```python
from build123d import *

# Parameters (mm, degrees)
SKETCH1_R           = 2.5
BOSS_EXTRUDE1_DEPTH = 3
SKETCH2_R           = 1.5
CUT_EXTRUDE1_DEPTH  = 77.127156728
FILLET1_R           = 10
SKETCH3_R           = 6
CUT_EXTRUDE2_DEPTH  = 77.127156728
BOSS_EXTRUDE3_DEPTH = 5
FILLET3_START       = -3.356502253
FILLET3_DEPTH       = 38.004734531
FILLET3_START_2     = -6
FILLET3_2_DEPTH     = 6


with BuildPart() as part:
    # Sketch1 → Boss-Extrude1 (new body)
    with BuildSketch(Plane.XY):
        with BuildLine():
            Line((0, -19), (30, -19))
            Line((30, -19), (64.201367261, 15.201367261))
            Line((64.201367261, 15.201367261), (58.615223689, 20.787510832))
            Line((58.615223689, 20.787510832), (44.190245353, 35.212489168))
            Line((44.190245353, 35.212489168), (38.604101782, 40.798632739))
            Line((38.604101782, 40.798632739), (16.805469042, 19))
            Line((16.805469042, 19), (0, 19))
            ThreePointArc((0, 19), (-19, 0), (0, -19))
        make_face()
        Circle(SKETCH1_R, mode=Mode.SUBTRACT)
    extrude(amount=BOSS_EXTRUDE1_DEPTH)

    # Sketch2 → Cut-Extrude1 (cut, through all)
    with BuildSketch(Plane.XY.offset(3)):
        with Locations((38.878105659, 35.574881393)):
            Circle(SKETCH2_R)
        with Locations((58.977615915, 15.475371138)):
            Circle(SKETCH2_R)
    extrude(amount=-CUT_EXTRUDE1_DEPTH, mode=Mode.SUBTRACT)

    # Fillet1
    fillet1_edges = [part.edges().sort_by_distance(p)[0] for p in [
        (16.805469042, 19, 1.5),
        (30, -19, 1.5),
    ]]
    fillet(fillet1_edges, radius=FILLET1_R)

    # Sketch3 → Cut-Extrude2 (cut, through all)
    with BuildSketch(Plane.XY.offset(3)):
        Circle(SKETCH3_R)
        Polygon((38.604101782, 40.798632739), (31.53303397, 33.727564928), (57.130299449, 8.130299449), (64.201367261, 15.201367261), align=None)
    extrude(amount=-CUT_EXTRUDE2_DEPTH, mode=Mode.SUBTRACT)

    # Sketch5 → Boss-Extrude3 (add)
    with BuildSketch(Plane(origin=(0, 0, 0), x_dir=(-1, 0, 0), z_dir=(0, 0, -1))):
        Polygon((-57.130299449, 8.130299449), (-31.53303397, 33.727564928), (-20.926432252, 23.12096321), (-46.523697731, -2.476302269), align=None)
    extrude(amount=BOSS_EXTRUDE3_DEPTH)

    # Fillet3: read off the stored shape, not the designer's step
    # Fillet3 outline → Fillet3 (add)
    with BuildSketch(Plane(origin=(0, 0, 0), x_dir=(0.707106781186548, 0.707106781186547, 0), z_dir=(0.707106781186547, -0.707106781186548, 0)).offset(FILLET3_START)):
        with BuildLine():
            ThreePointArc((23.730013537, 0), (28.202149492, -1.366750419), (31.146212025, -5))
            Line((31.146212025, -5), (31.146212025, 0))
            Line((31.146212025, 0), (23.730013537, 0))
        make_face()
    extrude(amount=FILLET3_DEPTH)

    # Fillet3 2 outline → Fillet3 2 (cut)
    with BuildSketch(Plane.XY.offset(FILLET3_START_2)):
        with BuildLine():
            Line((19.650292227, 24.397103235), (14.406247999, 19.153058913))
            ThreePointArc((14.406247999, 19.153058913), (17.283716467, 20.131400309), (19.73440123, 21.928932188))
            Line((19.73440123, 21.928932188), (20.926432252, 23.12096321))
            Line((20.926432252, 23.12096321), (19.650292227, 24.397103235))
        make_face()
    extrude(amount=FILLET3_2_DEPTH, mode=Mode.SUBTRACT)


solid = part.part
```
Model file for the job. Use its own axes, mm. A direction names the side the tool comes from. Coordinates: 2 decimals unless noted, no trailing zeros. Order: outer loops, then holes, each group sorted by start corner. A loop starts at its lowest first (then second) coordinate and runs counter-clockwise, first axis right, second up. Notation, with made-up numbers: (83.25, 3) -> (126.25, 3) arc R19 ccw to (126.25, 7) -> close; hole circle Ø4 at (29, 22). An arc over 180 degrees is marked (long way). Answer as a JSON object with one key per item and string values. Group by question number.
1) Cut at C-C, the plane z = -3.75. Write the cut outline in (x, y).
2) Pull direction X, two halves, no side cores. Call faces 3 (the face through (-6, 0, 2)), 4 (the face through (44.51, 20.75, -0.94)), 5 (the face through (11, 0, 0)), 6 (the face through (30.78, 9.03, -1.33)): +X half, -X half, draft (parallel to the pull), parting line (faces both ways), or undercut.
3) Which spindle directions (+Z, -Z, +X, -X, +Y, -Y) get a long thin tool onto all of the face, cutting with end or side? Do faces 1 (the face through (6, 19, 1)), 2 (the face through (-19, 0, 1)). Say none if no direction does.
4) Flat gauge pins, fed straight in: pin 1 (1.5 mm diameter, centred on y = 22, z = -2, fed in from +X); pin 2 (4 mm diameter, centred on y = 15, z = 0.5, fed in from -X); pin 3 (19 mm diameter, centred on x = 0, y = 7, fed in from -Z). Where does each tip first touch, or does it go through?
5) Cut at D-D, the plane y = 25. Write the cut outline in (x, z).
6) Drill centre lines: L1, parallel to Y at x = 0, z = 1.5; L2, parallel to Z at x = 19, y = -15.5; L3, parallel to Y at x = 12.5, z = 2. Where is each one in solid material? Low to high.
7) Cut at A-A, the plane x = 4. Write the cut outline in (y, z), then the cut area to 3 significant figures.
8) Cut at B-B, the plane y = 30.5. Write the cut outline in (x, z), then the cut area to 3 significant figures.
Check values:
{
 "1": {"outline": "(20.47, 22.67) -> (46.07, -2.93) -> (57.13, 8.13) -> (31.53, 33.73) -> close"},
 "2": {"face 3": "undercut", "face 4": "+X half", "face 5": "draft", "face 6": "-X half"},
 "3": {"face 1": "+Z, -Z, -X, +Y", "face 2": "+Z, -Z, -X"},
 "4": {"pin 1": "stops at x = 44.01", "pin 2": "stops at x = -13.86", "pin 3": "stops at z = 0"},
 "5": {"outline": "(22.81, -5) -> (40.26, -5) -> (40.26, 3) -> (22.81, 3) -> close"},
 "6": {"L1": "y = -19 to -6, 6 to 19", "L2": "z = 0 to 3", "L3": "y = -19 to 19"},
 "7": {"outline": "(-19, 0) -> (-4.47, 0) -> (-4.47, 3) -> (-19, 3) -> close; (4.47, 0) -> (19, 0) -> (19, 3) -> (4.47, 3) -> close", "area": "87.2 mm²"},
 "8": {"outline": "(28.31, -5) -> (34.76, -5) -> (34.76, 3) -> (28.31, 3) -> close", "area": "51.6 mm²"}
}
